```python
from build123d import *

# Parameters (mm, degrees)
NOTCH_180_SKETCH_W   = 18
NOTCH_180_SKETCH_H   = 19
NOTCH_180_DEPTH      = 4.175
NOTCH_225_DEPTH      = 4.175
NOTCH_270_SKETCH_W   = 19
NOTCH_270_SKETCH_H   = 18
NOTCH_270_DEPTH      = 4.175
SCREW_HOLE_SKETCH_W  = 1.65
SCREW_HOLE_SKETCH_H  = 9
SCREW_HOLES_X8_COUNT = 8


with BuildPart() as part:
    # Ring Sketch → Ring (revolve)
    with BuildSketch(Plane.XY, mode=Mode.PRIVATE) as ring_sk:
        Polygon((3.175, 70.5315), (3.175, 99), (-3.175, 99), (-3.175, 74.4685), align=None)
    revolve(ring_sk.sketch.rotate(Axis((-300, 0, 0), (1, 0, 0)), 90), axis=Axis((-300, 0, 0), (1, 0, 0)))

    # Notch 180 Sketch → Notch 180 (cut, symmetric)
    with BuildSketch(Plane(origin=(0, 0, 0), x_dir=(0, 0, -1), z_dir=(1, 0, 0))):
        with Locations((0, -91.5)):
            Rectangle(NOTCH_180_SKETCH_W, NOTCH_180_SKETCH_H)
    extrude(amount=NOTCH_180_DEPTH, both=True, mode=Mode.SUBTRACT)

    # Notch 225 Sketch → Notch 225 (cut, symmetric)
    with BuildSketch(Plane(origin=(0, 0, 0), x_dir=(0, 0, -1), z_dir=(1, 0, 0))):
        Polygon((51.618795027, -64.346717088), (64.346717088, -51.618795027), (77.781745931, -65.053823869), (65.053823869, -77.781745931), align=None)
    extrude(amount=NOTCH_225_DEPTH, both=True, mode=Mode.SUBTRACT)

    # Notch 270 Sketch → Notch 270 (cut, symmetric)
    with BuildSketch(Plane(origin=(0, 0, 0), x_dir=(0, 0, -1), z_dir=(1, 0, 0))):
        with Locations((91.5, 0)):
            Rectangle(NOTCH_270_SKETCH_W, NOTCH_270_SKETCH_H)
    extrude(amount=NOTCH_270_DEPTH, both=True, mode=Mode.SUBTRACT)

    # Screw Hole Sketch → Screw Hole (revolve, cut)
    with BuildSketch(Plane(origin=(0, 0, 0), x_dir=(-1, 0, 0), z_dir=(0, -0.3826834323650898, 0.9238795325112867)), mode=Mode.PRIVATE) as screw_hole_sk:
        with Locations((-0.825, -95.5)):
            Rectangle(SCREW_HOLE_SKETCH_W, SCREW_HOLE_SKETCH_H)
    screw_hole = revolve(screw_hole_sk.sketch.rotate(Axis((0, 81.301398861, 33.676142048), (0, 0.9238795325112867, 0.38268343236509)), 90), axis=Axis((0, 81.301398861, 33.676142048), (0, 0.9238795325112867, 0.38268343236509)), mode=Mode.SUBTRACT)

    # Screw Holes x8: Screw Hole ×8 about axis
    screw_holes_x8_axis = Axis((0, 0, 0), (1, 0, 0))
    for i in range(1, SCREW_HOLES_X8_COUNT):
        add(screw_hole.rotate(screw_holes_x8_axis, i * 360 / SCREW_HOLES_X8_COUNT), mode=Mode.SUBTRACT)


solid = part.part
```
Can you work these out from the model? Positions are in its coordinate system, mm. A direction names the side the tool comes from. Coordinates: 2 decimals unless noted, no trailing zeros. Order: outer loops, then holes, each group sorted by start corner. A loop starts at its lowest first (then second) coordinate and runs counter-clockwise, first axis right, second up. Notation, with made-up numbers: (44, -7) - (63, -7) arc R16 cw to (63, 10) - close; hole circle Ø4 at (2, -32). An arc over 180 degrees is marked (long way). Answer in a Markdown table with one row per item.
1. If I drill on line 1 along Z through (x, y) = (1, 36.5); line 2 along Y through (x, z) = (0, -10); line 3 along Z through (x, y) = (-2, 30), over which ranges is the centre line in solid material (lowest first)?
Reply:
| item | result |
|---|---|
| line 1 | z = -92.03 to -91.55, -84.69 to -61.92, 61.92 to 84.69, 91.55 to 92.03 |
| line 2 | y = -98.49 to -71.81, 71.81 to 98.49 |
| line 3 | z = -94.35 to -67.36, 67.36 to 94.35 |
2. Suppose I cut it at A-A (y = 0). Please give me the cut outline in (x, z) (1 decimal), and give its area (3 significant figures).
Reply:
| item | result |
|---|---|
| outline | (-3.2, -82) - (3.2, -82) - (3.2, -70.5) - (-3.2, -74.5) - close; (-3.2, 74.5) - (3.2, 70.5) - (3.2, 99) - (-3.2, 99) - close |
| area | 229 mm^2 |
3. For faces 1 (the flat face through (0, -82, 0)), 2 (the cylindrical face through (-0.496, -87.115, 37.788)), 3 (the flat face through (0, 9, -90)), which set-ups out of +Z, -Z, +X, -X, +Y, -Y let a thin tool reach every point of the face, with its end or its side?
Reply:
| item | result |
|---|---|
| face 1 | +X, -X, -Y |
| face 2 | none |
| face 3 | -Z, +X, -X |
4. If we mould it in two halves opening along X, with no side actions, what happens to faces 4 (the flat face through (0.044, -58.072, -57.894)), 5 (the cylindrical face through (-1.115, -87.252, -37.457)), 6 (the conical face through (2.867, -21.243, 67.457))? For each: pulls with the +X half, pulls with the -X half, needs draft (parallel to the pull), parting line crosses it, or undercut.
Reply:
| item | result |
|---|---|
| face 4 | needs draft |
| face 5 | undercut |
| face 6 | pulls with the -X half |
5. For pin 1 (3 mm diameter, centred on x = 2, z = 16.5, fed in from -Y); pin 2 (1.9 mm diameter, centred on x = 0.5, z = -89.5, fed in from -Y); pin 3 (2 mm diameter, centred on x = 0, z = 42.5, fed in from -Y), each with a flat end and sliding along its axis, tell me the tip position at first contact or that it passes through.
Reply:
| item | result |
|---|---|
| pin 1 | stops at y = -97.86 |
| pin 2 | stops at y = -44.27 |
| pin 3 | stops at y = -89.88 |
